from build123d import *

# Parameters (mm, degrees)
BOSS_EXTRUDE1_DEPTH = 1
FILLET2_R           = 4.8
SKETCH5_W           = 29
SKETCH5_H           = 0.8
BOSS_EXTRUDE2_DEPTH = 1
CUT_EXTRUDE1_REACH  = 105.527
CIRPATTERN1_COUNT   = 4
SKETCH6_R           = 23.9
SKETCH6_R_2         = 21.9
BOSS_EXTRUDE3_DEPTH = 16
FILLET6_R           = 2
CHAMFER1_SIZE       = 1
FILLET5_R           = 2
FILLET7_R           = 0.5


with BuildPart() as part:
    # Sketch4 → Boss-Extrude1 (new body)
    with BuildSketch(Plane(origin=(0, 0, 0), x_dir=(1, 0, 0), z_dir=(0, 1, 0))):
        with BuildLine():
            Line((72.8, -27.525603906), (72.8, 27.525603906))
            ThreePointArc((72.8, 27.525603906), (68.286783321, 28.285311783), (70.940914849, 32.013832492))
            Line((70.940914849, 32.013832492), (32.013832492, 70.940914849))
            ThreePointArc((32.013832492, 70.940914849), (28.285311783, 68.286783321), (27.525603906, 72.8))
            Line((27.525603906, 72.8), (-27.525603906, 72.8))
            ThreePointArc((-27.525603906, 72.8), (-28.285311783, 68.286783321), (-32.013832492, 70.940914849))
            Line((-32.013832492, 70.940914849), (-70.940914849, 32.013832492))
            ThreePointArc((-70.940914849, 32.013832492), (-68.286783321, 28.285311783), (-72.8, 27.525603906))
            Line((-72.8, 27.525603906), (-72.8, -27.525603906))
            ThreePointArc((-72.8, -27.525603906), (-68.286783321, -28.285311783), (-70.940914849, -32.013832492))
            Line((-70.940914849, -32.013832492), (-32.013832492, -70.940914849))
            ThreePointArc((-32.013832492, -70.940914849), (-28.285311783, -68.286783321), (-27.525603906, -72.8))
            Line((-27.525603906, -72.8), (27.525603906, -72.8))
            ThreePointArc((27.525603906, -72.8), (28.285311783, -68.286783321), (32.013832492, -70.940914849))
            Line((32.013832492, -70.940914849), (70.940914849, -32.013832492))
            ThreePointArc((70.940914849, -32.013832492), (68.286783321, -28.285311783), (72.8, -27.525603906))
        make_face()
    extrude(amount=BOSS_EXTRUDE1_DEPTH)

    # Fillet2
    fillet2_edges = [part.edges().sort_by_distance(p)[0] for p in [
        (27.525603906, 0.5, 72.8),
        (-27.525603906, 0.5, 72.8),
        (-32.013832492, 0.5, 70.940914849),
        (-70.940914849, 0.5, 32.013832492),
        (-72.8, 0.5, 27.525603906),
        (-72.8, 0.5, -27.525603906),
        (-70.940914849, 0.5, -32.013832492),
        (-32.013832492, 0.5, -70.940914849),
        (-27.525603906, 0.5, -72.8),
        (27.525603906, 0.5, -72.8),
        (32.013832492, 0.5, -70.940914849),
        (70.940914849, 0.5, -32.013832492),
        (72.8, 0.5, -27.525603906),
        (72.8, 0.5, 27.525603906),
        (70.940914849, 0.5, 32.013832492),
        (32.013832492, 0.5, 70.940914849),
    ]]
    fillet(fillet2_edges, radius=FILLET2_R)

    # Sketch5 → Boss-Extrude2 (add)
    with BuildSketch(Plane(origin=(0, 1, 0), x_dir=(1, 0, 0), z_dir=(0, 1, 0))):
        with Locations((0, 73.2)):
            Rectangle(SKETCH5_W, SKETCH5_H)
    boss_extrude2 = extrude(amount=-BOSS_EXTRUDE2_DEPTH)

    # Sketch7 → Cut-Extrude1 (cut, up to next)
    with BuildSketch(Plane(origin=(0, 1, 0), x_dir=(1, 0, 0), z_dir=(0, 1, 0)), mode=Mode.PRIVATE) as cut_extrude1_sk1:
        with BuildLine():
            Line((58.548441482, 44.406305859), (44.406305859, 58.548441482))
            ThreePointArc((44.406305859, 58.548441482), (44.406305859, 44.406305859), (58.548441482, 44.406305859))
        make_face()
    cut_extrude1_tool1 = extrude(cut_extrude1_sk1.sketch, amount=-CUT_EXTRUDE1_REACH, mode=Mode.PRIVATE) & part.part
    cut_extrude1 = cut_extrude1_tool1.solids().sort_by_distance((48.476319, 1, -48.476319))[0]
    add(cut_extrude1, mode=Mode.SUBTRACT)

    # CirPattern1: Boss-Extrude2, Cut-Extrude1 ×4 about axis
    cirpattern1_axis = Axis((0, 0, 0), (0, 1, 0))
    add([boss_extrude2.rotate(cirpattern1_axis, i * 360 / CIRPATTERN1_COUNT) for i in range(1, CIRPATTERN1_COUNT)])
    add([cut_extrude1.rotate(cirpattern1_axis, i * 360 / CIRPATTERN1_COUNT) for i in range(1, CIRPATTERN1_COUNT)], mode=Mode.SUBTRACT)

    # Sketch6 → Boss-Extrude3 (add)
    with BuildSketch(Plane(origin=(0, 1, 0), x_dir=(1, 0, 0), z_dir=(0, 1, 0))):
        with Locations(Location((0, 0, 0), (0, 0, 270))):
            Circle(SKETCH6_R)
        with Locations(Location((0, 0, 0), (0, 0, 270))):
            Circle(SKETCH6_R_2, mode=Mode.SUBTRACT)
    extrude(amount=BOSS_EXTRUDE3_DEPTH)

    # Fillet6
    fillet6_edges = [part.edges().sort_by_distance(p)[0] for p in [
        (58.548441482, 0.5, -44.406305859),
        (44.406305859, 0.5, -58.548441482),
        (44.406305859, 0.5, 58.548441482),
        (58.548441482, 0.5, 44.406305859),
        (-58.548441482, 0.5, 44.406305859),
        (-44.406305859, 0.5, 58.548441482),
        (-44.406305859, 0.5, -58.548441482),
        (-58.548441482, 0.5, -44.406305859),
    ]]
    fillet(fillet6_edges, radius=FILLET6_R)

    # Chamfer1
    chamfer1_edges = [part.edges().sort_by_distance(p)[0] for p in [
        (0, 17, -21.9),
    ]]
    chamfer(chamfer1_edges, length=CHAMFER1_SIZE)

    # Fillet5
    fillet5_edges = [part.edges().sort_by_distance(p)[0] for p in [
        (0, 1, -21.9),
        (0, 1, -23.9),
    ]]
    fillet(fillet5_edges, radius=FILLET5_R)

    # Fillet7
    fillet7_edges = [part.edges().sort_by_distance(p)[0] for p in [
        (-14.5, 0.5, -73.6),
        (14.5, 0.5, -73.6),
        (73.6, 0.5, -14.5),
        (73.6, 0.5, 14.5),
        (14.5, 0.5, 73.6),
        (-14.5, 0.5, 73.6),
        (-73.6, 0.5, 14.5),
        (-73.6, 0.5, -14.5),
    ]]
    fillet(fillet7_edges, radius=FILLET7_R)


solid = part.part
The listing builds one solid part. Answer for the finished solid, in the listing's coordinates (mm). A direction names the side the tool comes from. Give positions to 0.01 mm unless a question says otherwise; leave off trailing zeros. Loops run counter-clockwise (first coordinate to the right, second up) from the corner with the lowest first, then second, coordinate; pieces in that order, holes last.
Item 1: A cutting plane is placed at B-B (x = 0). Give the vertices of the cut face in (y, z).
Derived:
outline: (0, -73.6) - (1, -73.6) - (1, -25.9) arc R2 cw to (3, -23.9) - (17, -23.9) - (17, -22.9) - (16, -21.9) - (3, -21.9) arc R2 cw to (1, -19.9) - (1, 19.9) arc R2 cw to (3, 21.9) - (16, 21.9) - (17, 22.9) - (17, 23.9) - (3, 23.9) arc R2 cw to (1, 25.9) - (1, 73.6) - (0, 73.6) - close
Item 2: A cutting plane is placed at A-A (z = 0). Give the vertices of the cut face in (x, y).
Derived:
outline: (-73.6, 0) - (73.6, 0) - (73.6, 1) - (25.9, 1) arc R2 cw to (23.9, 3) - (23.9, 17) - (22.9, 17) - (21.9, 16) - (21.9, 3) arc R2 cw to (19.9, 1) - (-19.9, 1) arc R2 cw to (-21.9, 3) - (-21.9, 16) - (-22.9, 17) - (-23.9, 17) - (-23.9, 3) arc R2 cw to (-25.9, 1) - (-73.6, 1) - close
Item 3: A cutting plane is placed at D-D (z = 45.5). Give the vertices of the cut face in (x, y).
Derived:
outline: (-43.46, 0) - (43.46, 0) - (43.46, 1) - (-43.46, 1) - close
Item 4: Find the intervals of material crossed by line 1 along X through (y, z) = (5.5, 0); line 2 along Y through (x, z) = (-12, -5.5); line 3 along Z through (x, y) = (-20, 15), in increasing order.
Derived:
line 1: x = -23.9 to -21.9, 21.9 to 23.9
line 2: y = 0 to 1
line 3: z = -13.08 to -8.92, 8.92 to 13.08
Item 5: A tool of negligible diameter and unlimited length cuts with its end or side. For faces 1 (the flat face through (-23, 17, 2)), 2 (the flat face through (0, 1, 0)), from which of +Z, -Z, +X, -X, +Y, -Y can it reach the whole face along a straight path? Write none if from no direction.
Derived:
face 1: +Z, -Z, +X, -X, +Y
face 2: +Y
Item 6: Each of these flat-tipped pins is pushed along its axis until it touches: pin 1 Ø1.1 at (y, z) = (0.5, 17.5) entering from +X; pin 2 Ø5 at (x, z) = (-56, -7) entering from +Y; pin 3 Ø10 at (x, z) = (-53, -58) entering from -Y; pin 4 Ø0.5 at (x, y) = (20, 0.5) entering from +Z. Where does it stop, or does it pass through?
Derived:
pin 1: stops at x = 72.8
pin 2: stops at y = 1
pin 3: passes through
pin 4: stops at z = 72.8
Item 7: Determine the mould class of faces 3 (the flat face through (63.512, 0.493, 39.443)), 4 (the cylindrical face through (6.58, 9.41, 20.89)), 5 (the flat face through (32, 1, -1)), 6 (the cylindrical face through (44.269, 0.507, -44.547)) for opening direction Z: +Z half, -Z half, draft (parallel to the pull), parting line (faces both ways), or undercut.
Derived:
face 3: +Z half
face 4: undercut
face 5: draft
face 6: undercut
Item 8: A cutting plane is placed at C-C (y = 13). Give the vertices of the cut face in (x, z).
Derived:
outline: circle Ø47.8 at (0, 0); hole circle Ø43.8 at (0, 0)
